Here's how the part is built. I have some questions about the finished solid (model axes, mm). A direction names the side the tool comes from. Coordinates: 2 decimals unless noted, no trailing zeros. Write each loop counter-clockwise with the first axis right and the second up, starting at its lowest first coordinate (ties: lowest second). Pieces come first, ordered by that corner, then holes.
Item 1: Please list where these lines run through material, in increasing order: line 1 (Y direction, x = -16, z = 3.35); line 2 (X direction, y = 12.75, z = 2.7).
Item 2: I want a section at C-C (y = 11). Please give me the cut outline in (x, z), and give its area (3 significant figures).
Item 3: I want a section at B-B (x = -16.5). Please give me the cut outline in (y, z), and give its area (3 significant figures).
Item 4: For faces 1 (the face through (-10, 7, 2)), 2 (the face through (10, 8, 2)), 3 (the face through (0, 15, 4)), which set-ups out of +Z, -Z, +X, -X, +Y, -Y let a thin tool reach every point of the face, with its end or its side?
Item 5: I'm going to push flat-ended pins straight in: P1, Ø1.2, axis at y = 5, z = 2.5, coming from the -X side; P2, Ø2, axis at x = 14.5, z = 1.5, coming from the -Y side; P3, Ø1, axis at x = -10, y = 8.5, coming from the -Z side; P4, Ø2, axis at y = 6.5, z = 1, coming from the +X side. Where does each tip first touch, or does it pass through?
Item 6: I want a section at A-A (z = 2.3). Please give me the cut outline in (x, y).
Autodesk Inventor part; units mm, degrees
ref_plane "YZ Plane" through (0, 0, 0) normal (1, 0, 0) x (0, 1, 0)
ref_plane "XZ Plane" through (0, 0, 0) normal (0, 1, 0) x (-1, 0, 0)
ref_plane "XY Plane" through (0, 0, 0) normal (0, 0, 1) x (1, 0, 0)
sketch "Sketch1" plane through (0, 0, 0) normal (0, 0, 1) x (1, 0, 0)
  line L0 (10, 0) -> (-10, 0)
  line L1 (-10, 0) -> (-10, 15)
  line L2 (-10, 15) -> (10, 15)
  line L3 (10, 15) -> (10, 0)
  line L4 (25, 15) -> (-25, 15)
  line L5 (-25, 15) -> (-25, 25)
  line L6 (-25, 25) -> (25, 25)
  line L7 (25, 25) -> (25, 15)
  point P0 (0, 0)
  point P1 (0, 0)
  point P2 (0, 15)
  point P3 (0, 15)
  point P4 (10, 15)
  dimension "d0" = 20
  dimension "d1" = 15
  dimension "d2" = 10
  dimension "d3" = 50
extrude "Extrusion1" add sketch "Sketch1" along normal blind 4
properties part number "Seguro"
Answer:
1. line 1: y = 15 to 25
1. line 2: x = -10 to 10
2. outline: (-10, 0) - (10, 0) - (10, 4) - (-10, 4) - close
2. area: 80.0 mm2
3. outline: (15, 0) - (25, 0) - (25, 4) - (15, 4) - close
3. area: 40.0 mm2
4. face 1: +Z, -Z, -X, -Y
4. face 2: +Z, -Z, +X, -Y
4. face 3: +Z, +X, -X, +Y, -Y
5. P1: stops at x = -10
5. P2: stops at y = 15
5. P3: stops at z = 0
5. P4: stops at x = 10
6. outline: (-25, 15) - (-10, 15) - (-10, 0) - (10, 0) - (10, 15) - (25, 15) - (25, 25) - (-25, 25) - close
